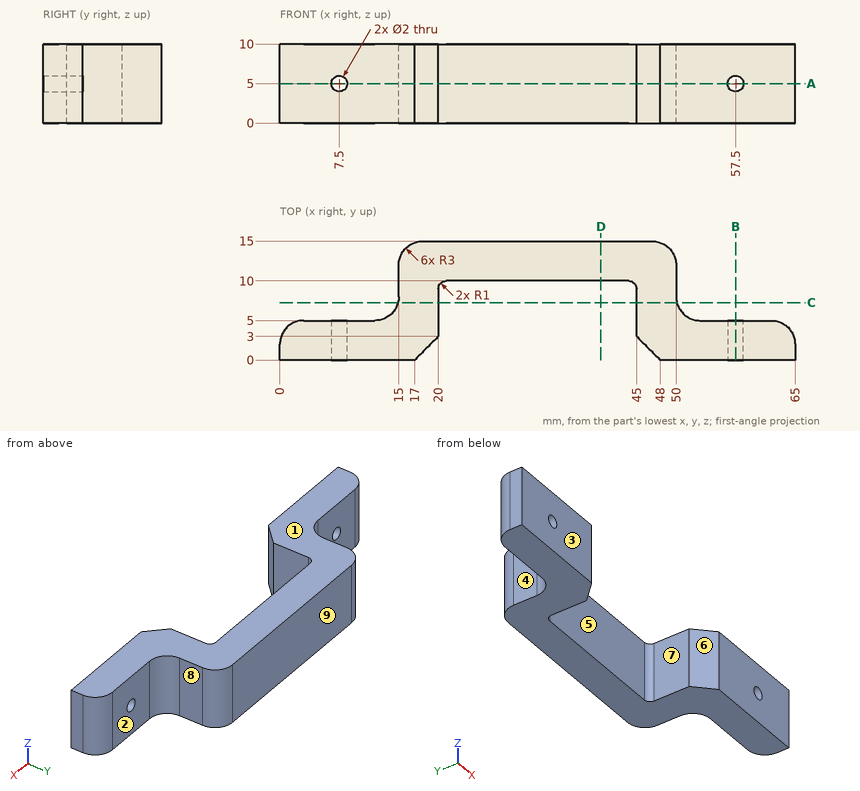
Here's the drawing with two shaded views (mm, measured from the low corner). I have some questions. A direction names the side the tool comes from. Coordinates: 2 decimals unless noted, no trailing zeros. Loops run counter-clockwise (first coordinate to the right, second up) from the corner with the lowest first, then second, coordinate; pieces in that order, holes last. Notation, with made-up numbers: (6.25, 30) -> (40.25, 30) arc R26 cw to (40.25, 65) -> close; hole circle Ø3 at (21, 10.25). An arc over 180 degrees is marked (long way). Put each result on its own line as item: value. Start each with the question number.
Q1. I want a section at A-A (z = 5). Count the separate pieces of the cut face and the enclosed holes in it, plus the area to 3 significant figures.
Q2. Thinking about a two-plate mould opening in X: for the marked faces 6, 7, 8 and 9, which applies, pulls with the +X half, pulls with the -X half, needs draft (parallel to the pull), parting line crosses it, or undercut?
Q3. I want a section at C-C (y = 7.25). Write out the boundary of the cut face in (x, z).
Q4. I want a section at B-B (x = 57.5). Write out the boundary of the cut face in (y, z).
Q5. If I drill on line 1 (X direction, y = 11.75, z = 9); line 2 (X direction, y = 9, z = 7); line 3 (Y direction, x = 21, z = 6.5), over which ranges is the centre line in solid material (lowest first)? Write a range as [from, to].
Q6. For the marked faces 1, 2, 3, 4 and 5, which set-ups out of +Z, -Z, +X, -X, +Y, -Y let a thin tool reach every point of the face, with its end or its side?
Q7. I'm going to push flat-ended pins straight in: P1, Ø1.8, axis at x = 57.5, z = 5, coming from the -Y side; P2, Ø2, axis at y = 10.5, z = 7, coming from the +X side; P3, Ø1.5, axis at x = 33, z = 5, coming from the -Y side; P4, Ø5, axis at y = 5.5, z = 6.5, coming from the -X side. Where does each tip first touch, or does it pass through?
Q8. I want a section at D-D (x = 40.5). Write out the boundary of the cut face in (y, z).
Taken from the geometry:
1. separate pieces: 3
1. enclosed holes: 0
1. area: 393 mm2
2. face 6: undercut
2. face 7: undercut
2. face 8: pulls with the +X half
2. face 9: needs draft
3. outline: (14.9, 0) -> (20, 0) -> (20, 10) -> (14.9, 10) -> close; (45, 0) -> (50.1, 0) -> (50.1, 10) -> (45, 10) -> close
4. outline: (0, 0) -> (5, 0) -> (5, 4) -> (0, 4) -> close; (0, 6) -> (5, 6) -> (5, 10) -> (0, 10) -> close
5. line 1: x = [15, 50]
5. line 2: x = [15, 20], [45, 50]
5. line 3: y = [10, 15]
6. face 1: +Z, +X, -X, +Y, -Y
6. face 2: +Z, -Z, +X, +Y
6. face 3: +Z, -Z, +X, -X, -Y
6. face 4: +Z, -Z, -X, +Y
6. face 5: +Z, -Z, -Y
7. P1: passes through
7. P2: stops at x = 50
7. P3: stops at y = 10
7. P4: stops at x = 0.17
8. outline: (10, 0) -> (15, 0) -> (15, 10) -> (10, 10) -> close
